The listing builds one solid part. Answer for the finished solid, in the listing's coordinates (mm). Face numbers are marked on the shaded views. A direction names the side the tool comes from. Coordinates: 2 decimals unless noted, no trailing zeros. Loops run counter-clockwise (first coordinate to the right, second up) from the corner with the lowest first, then second, coordinate; pieces in that order, holes last. Notation, with made-up numbers: (83, 24) -> (88, 24) arc R11 ccw to (88, 44) -> close; hole circle Ø3 at (6.25, -13.5). An arc over 180 degrees is marked (long way). Answer in a Markdown table with one row per item.
```python
from build123d import *

# Parameters (mm, degrees)
F1_DEPTH    = 51
F2_T1_DEPTH = 102.5
F2_T3_DEPTH = 102.5
F2_T6_ANGLE = 180
F2_T8_ANGLE = 180
F3_T        = -2.5


# Not quite as in the source:
# - a fillet or chamfer that OpenCascade refuses, or shapes differently, is made with other operations: its cross-section is extruded or revolved along the edge and cut away or added


with BuildPart() as f1:
    # F0 (on Top) → F1 (new body)
    with BuildSketch(Plane.XY):
        with BuildLine():
            Line((-70, 37.5), (-70, -37.5))
            Line((-70, -37.5), (-5, -37.5))
            ThreePointArc((-5, -37.5), (-3.5355339059, -33.9644660941), (0, -32.5))
            Line((0, -32.5), (0, 0))
            Line((0, 0), (0, 32.5))
            ThreePointArc((0, 32.5), (-3.5355339059, 33.9644660941), (-5, 37.5))
            Line((-5, 37.5), (-70, 37.5))
        make_face()
        with BuildLine():
            ThreePointArc((-70, 37.5), (-107.5, 0), (-70, -37.5))
            Line((-70, -37.5), (-70, 37.5))
        make_face()
        with BuildLine():
            Line((0, 0), (0, -32.5))
            ThreePointArc((0, -32.5), (3.5355339059, -33.9644660941), (5, -37.5))
            Line((5, -37.5), (70, -37.5))
            Line((70, -37.5), (70, 37.5))
            Line((70, 37.5), (5, 37.5))
            ThreePointArc((5, 37.5), (3.5355339059, 33.9644660941), (0, 32.5))
            Line((0, 32.5), (0, 0))
        make_face()
        with BuildLine():
            Line((70, 37.5), (70, -37.5))
            ThreePointArc((70, -37.5), (107.5, 0), (70, 37.5))
        make_face()
    extrude(amount=F1_DEPTH)

    # F2: fillet of radius 15 on 6 edges, made by hand

    # F2_s2 → F2_t1 (cut)
    with BuildSketch(Plane.YZ.offset(-32.5)):
        with BuildLine():
            ThreePointArc((-37.5, 36), (-33.1066017178, 46.6066017178), (-22.5, 51))
            Line((-22.5, 51), (-37.5, 51))
            Line((-37.5, 51), (-37.5, 36))
        make_face()
        with BuildLine():
            ThreePointArc((37.5, 36), (33.1066017178, 46.6066017178), (22.5, 51))
            Line((22.5, 51), (37.5, 51))
            Line((37.5, 51), (37.5, 36))
        make_face()
    extrude(amount=F2_T1_DEPTH, mode=Mode.SUBTRACT)

    # F2_s4 → F2_t3 (cut)
    with BuildSketch(Plane.YZ.offset(-70)):
        with BuildLine():
            ThreePointArc((37.5, 36), (33.1066017178, 46.6066017178), (22.5, 51))
            Line((22.5, 51), (37.5, 51))
            Line((37.5, 51), (37.5, 36))
        make_face()
        with BuildLine():
            ThreePointArc((-37.5, 36), (-33.1066017178, 46.6066017178), (-22.5, 51))
            Line((-22.5, 51), (-37.5, 51))
            Line((-37.5, 51), (-37.5, 36))
        make_face()
    extrude(amount=F2_T3_DEPTH, mode=Mode.SUBTRACT)

    # F2_s5 → F2_t6 (revolve, cut)
    with BuildSketch(Plane.YZ.offset(70)):
        with BuildLine():
            ThreePointArc((-37.5, 36), (-33.1066017178, 46.6066017178), (-22.5, 51))
            Line((-22.5, 51), (-37.5, 51))
            Line((-37.5, 51), (-37.5, 36))
        make_face()
    revolve(axis=Axis((70, 0, 51), (0, 0, 1)), revolution_arc=F2_T6_ANGLE, mode=Mode.SUBTRACT)

    # F2_s7 → F2_t8 (revolve, cut)
    with BuildSketch(Plane.YZ.offset(-70)):
        with BuildLine():
            ThreePointArc((37.5, 36), (33.1066017178, 46.6066017178), (22.5, 51))
            Line((22.5, 51), (37.5, 51))
            Line((37.5, 51), (37.5, 36))
        make_face()
    revolve(axis=Axis((-70, 0, 51), (0, 0, 1)), revolution_arc=F2_T8_ANGLE, mode=Mode.SUBTRACT)

    # F3
    f3_openings = [f1.faces().sort_by_distance(p)[0] for p in [
        (0, 0, 0),
    ]]
    offset(amount=F3_T, openings=f3_openings)


solid = f1.part
```
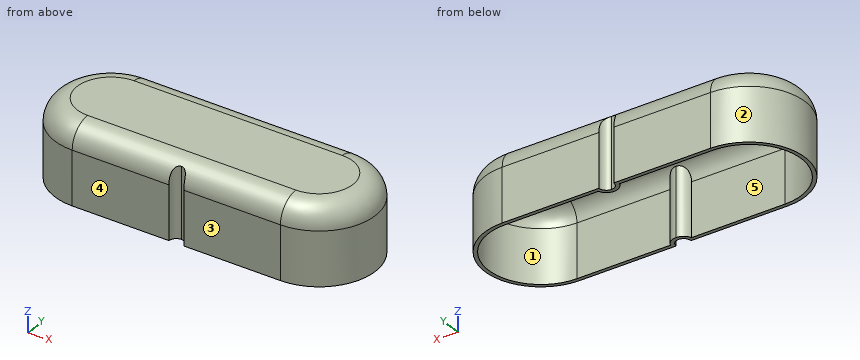
Item 1: A cutting plane is placed at A-A, the plane x = 34.5. Determine the outline of the cut face in (y, z), plus the area to 3 significant figures.
Findings below:
| item | result |
|---|---|
| outline | (-37.5, 0) -> (-35, 0) -> (-35, 36) arc R12.5 cw to (-22.5, 48.5) -> (22.5, 48.5) arc R12.5 cw to (35, 36) -> (35, 0) -> (37.5, 0) -> (37.5, 36) arc R15 ccw to (22.5, 51) -> (-22.5, 51) arc R15 ccw to (-37.5, 36) -> close |
| area | 400 mm2 |
Item 2: A cutting plane is placed at C-C, the plane y = 0. Determine the outline of the cut face in (x, z), plus the area to 3 significant figures.
Findings below:
| item | result |
|---|---|
| outline | (-107.5, 0) -> (-105, 0) -> (-105, 36) arc R12.5 cw to (-92.5, 48.5) -> (92.5, 48.5) arc R12.5 cw to (105, 36) -> (105, 0) -> (107.5, 0) -> (107.5, 36) arc R15 ccw to (92.5, 51) -> (-92.5, 51) arc R15 ccw to (-107.5, 36) -> close |
| area | 750 mm2 |
Item 3: Determine the mould class of the marked faces 1, 2 and 3 for opening direction X: +X half, -X half, draft (parallel to the pull), parting line (faces both ways), or undercut.
Findings below:
| item | result |
|---|---|
| face 1 | undercut |
| face 2 | -X half |
| face 3 | draft |
Item 4: Find the intervals of material crossed by probe 1 along Y at (x, z) = (36.5, 22); probe 2 along Z at (x, y) = (-49.5, 15); probe 3 along X at (y, z) = (-12, 46), in increasing order.
Findings below:
| item | result |
|---|---|
| probe 1 | y = -37.5 to -35, 35 to 37.5 |
| probe 2 | z = 48.5 to 51 |
| probe 3 | x = -101.47 to -97.5, 97.5 to 101.47 |
Item 5: A tool of negligible diameter and unlimited length cuts with its end or side. For the marked faces 4 and 5, from which of +Z, -Z, +X, -X, +Y, -Y can it reach the whole face along a straight path? Write none if from no direction.
Findings below:
| item | result |
|---|---|
| face 4 | +Z, -Z, +X, -X, -Y |
| face 5 | -Z |
Item 6: A cutting plane is placed at D-D, the plane z = 39.5. Determine the outline of the cut face in (x, y).
Findings below:
| item | result |
|---|---|
| outline | (-70, -37.09) -> (-4.98, -37.09) arc R5 cw to (4.98, -37.09) -> (70, -37.09) arc R37.09 ccw to (70, 37.09) -> (4.98, 37.09) arc R5 cw to (-4.98, 37.09) -> (-70, 37.09) arc R37.09 ccw to start; hole (-70, -34.5) -> (-6.87, -34.5) arc R7.5 cw to (6.87, -34.5) -> (70, -34.5) arc R34.5 ccw to (70, 34.5) -> (6.87, 34.5) arc R7.5 cw to (-6.87, 34.5) -> (-70, 34.5) arc R34.5 ccw to start |
Item 7: Flat-ended cylindrical pins translate along their axes: pin 1 Ø8 at (y, z) = (27.5, 5.5) entering from +X; pin 2 Ø10 at (y, z) = (10, 37.5) entering from -X; pin 3 Ø6 at (x, y) = (-8, 28) entering from +Z. Find the tip coordinate at first contact, or state that the pin passes through.
Findings below:
| item | result |
|---|---|
| pin 1 | stops at x = 99.22 |
| pin 2 | stops at x = -107.14 |
| pin 3 | stops at z = 50.79 |
Item 8: A cutting plane is placed at B-B, the plane z = 7.5. Determine the outline of the cut face in (x, y).
Findings below:
| item | result |
|---|---|
| outline | (-70, -37.5) -> (-5, -37.5) arc R5 cw to (5, -37.5) -> (70, -37.5) arc R37.5 ccw to (70, 37.5) -> (5, 37.5) arc R5 cw to (-5, 37.5) -> (-70, 37.5) arc R37.5 ccw to start; hole (-70, -35) -> (-7.07, -35) arc R7.5 cw to (7.07, -35) -> (70, -35) arc R35 ccw to (70, 35) -> (7.07, 35) arc R7.5 cw to (-7.07, 35) -> (-70, 35) arc R35 ccw to start |
